Can you work these out from the model? Positions are in its coordinate system, mm. Face numbers are marked on the shaded views. A direction names the side the tool comes from. Give positions to 0.01 mm unless a question says otherwise; leave off trailing zeros. Write each loop counter-clockwise with the first axis right and the second up, starting at its lowest first coordinate (ties: lowest second). Pieces come first, ordered by that corner, then holes. Notation, with made-up numbers: M 18,35 L 39,35 A30 ccw 39,60 Z; hole C -18.75,38.25 d3. An arc over 180 degrees is marked long. Write each question's results on one line, items separated by ' | '.
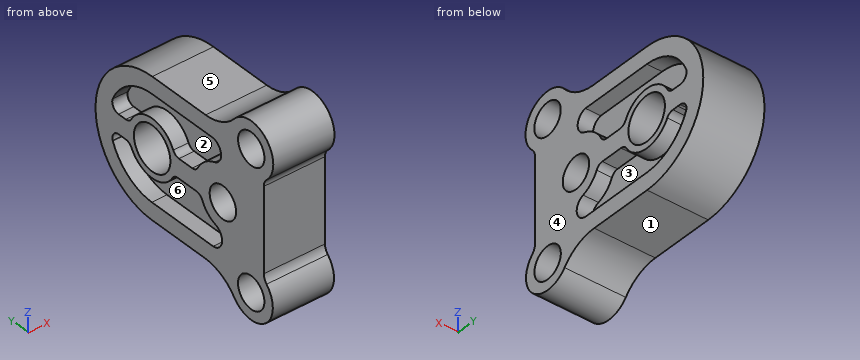
Autodesk Inventor part; units mm, degrees
ref_plane "YZ Plane" through (0, 0, 0) normal (1, 0, 0) x (0, 1, 0)
ref_plane "XZ Plane" through (0, 0, 0) normal (0, 1, 0) x (-1, 0, 0)
ref_plane "XY Plane" through (0, 0, 0) normal (0, 0, 1) x (1, 0, 0)
sketch "Sketch1" plane through (0, 0, 0) normal (1, 0, 0) x (0, 1, 0)
  arc A0 (176.1097, -208.7052) -> (175.3048, -28.7073) centre (175.5363, -118.707) ccw
  line L0 (175.3048, -28.7073) -> (90.5303, -28.7073)
  line L1 (-1.9186, -65.845) -> (-1.9186, -175.1547)
  line L2 (92.0444, -208.7052) -> (176.1097, -208.7052)
  arc A1 (44.7113, -7.4451) -> (-6.4479, -55.1041) centre (17.9836, -30.0422) ccw
  arc A2 (-6.3181, -185.8489) -> (45.0423, -231.4117) centre (18.1097, -210.0421) ccw
  line L3 (175.7375, -50.7073) -> (78.1247, -50.7073)
  line L4 (133.0218, -107.5228) -> (111.9726, -107.5228)
  line L5 (105.0926, -132.5228) -> (134.6019, -132.5228)
  arc A3 (208.5623, -100.9438) -> (141.9722, -101.9826) centre (175.5363, -118.707) ccw
  arc A4 (103.0885, -102.1131) -> (76.4229, -79.7842) centre (63.1097, -122.7698) ccw
  arc A5 (74.6044, -157.3047) -> (96.0441, -138.2655) centre (63.1097, -122.7698) ccw
  circle A6 centre (63.1097, -122.7698) radius 21
  circle A7 centre (17.9836, -30.0422) radius 21
  circle A8 centre (18.1097, -210.0421) radius 21
  arc A9 (44.7113, -7.4451) -> (90.5303, -28.7073) centre (90.5303, 31.2927) ccw
  arc A10 (92.0444, -208.7052) -> (45.0423, -231.4117) centre (92.0444, -268.7052) ccw
  arc A11 (-1.9186, -65.845) -> (-6.4479, -55.1041) centre (-16.9186, -65.845) ccw
  arc A12 (-6.3181, -185.8489) -> (-1.9186, -175.1547) centre (-17.1159, -175.1547) ccw
  arc A13 (78.1247, -50.7073) -> (76.4229, -79.7842) centre (80.8606, -65.4557) ccw
  arc A14 (74.6044, -157.3047) -> (78.6837, -186.5226) centre (79.3415, -171.5371) ccw
  circle A15 centre (175.5363, -118.707) radius 29
  arc A16 (133.0218, -107.5228) -> (141.9722, -101.9826) centre (133.0218, -97.5228) ccw
  arc A17 (143.2454, -137.4939) -> (134.6019, -132.5228) centre (134.6019, -142.5228) ccw
  arc A18 (103.0885, -102.1131) -> (111.9726, -107.5228) centre (111.9726, -97.5228) ccw
  arc A19 (105.0926, -132.5228) -> (96.0441, -138.2655) centre (105.0926, -142.5228) ccw
  line L6 (217.3693, -106.207) -> (225.3783, -106.207)
  line L7 (225.3783, -106.207) -> (229.2504, -106.207)
  line L8 (225.1161, -131.2646) -> (228.7337, -131.2481)
  line L9 (228.7337, -131.2481) -> (217.1089, -131.3029)
  arc A20 (217.1089, -131.3029) -> (208.3269, -136.6074) centre (217.156, -141.3028) ccw
  arc A21 (208.5623, -100.9438) -> (217.3693, -106.207) centre (217.3693, -96.207) ccw
  line L10 (119.8472, -132.5228) -> (119.8472, -186.8276)
  arc A22 (176.0639, -186.5226) -> (238.0141, -145.0843) centre (175.5363, -118.707) ccw
  arc A23 (143.2454, -137.4939) -> (208.3269, -136.6074) centre (175.5363, -118.707) ccw
  line L11 (176.0639, -186.5226) -> (78.6837, -186.5226)
  arc A24 (238.2111, -92.3277) -> (175.7375, -50.7073) centre (175.5363, -118.707) ccw
  line L12 (229.2504, -106.207) -> (228.9942, -106.207)
  arc A25 (228.9942, -106.207) -> (238.2111, -92.3277) centre (228.9942, -96.207) ccw
  line L13 (228.7337, -131.2481) -> (228.7379, -131.2481)
  line L14 (238.2764, -144.2509) -> (238.0141, -145.0843)
  arc A26 (238.2764, -144.2509) -> (228.7379, -131.2481) centre (228.7379, -141.2481) ccw
  point P0 (0, 0)
  point P1 (0, 0)
  point P2 (-1.9186, -182.0976)
  point P3 (139.7429, -107.5228)
  point P4 (140.8602, -132.5228)
  point P5 (105.4479, -107.5228)
  point P6 (98.1763, -132.5228)
  point P7 (-1.9186, -58.8329)
  point P8 (210.8916, -106.207)
  point P9 (242.3775, -106.207)
  dimension "d36" = 60
  dimension "d37" = 42
  dimension "d38" = 35
  dimension "d40" = 42
  dimension "d41" = 45
  dimension "d42" = 45
  dimension "d50" = 90
  dimension "d51" = 15
  dimension "d52" = 15
  dimension "d53" = 15
  dimension "d54" = 180
  dimension "d55" = 60
  dimension "d64" = 58
  dimension "d66" = 25
  dimension "d68" = 10
  dimension "d69" = 37.5
  dimension "d75" = 22
  dimension "d79" = 10
extrude "Extrusion1" add sketch "Sketch1" along normal blind 40 and the other way blind 40
sketch "Sketch2" plane through (40, 0, 0) normal (1, 0, 0) x (0, 0, -1)
  point P0 (0, 0)
extrude "Extrusion2" add sketch "Sketch1" along normal blind 20 and the other way blind 20 contours A24 A25 L7 L6 A21 A3 A16 L4 A18 A4 A13 L3 | L5 L10 L11 A14 A5 A19 | L5 A17 A23 A20 L9 L8 L13 A26 L14 A22 L11 L10
properties part number "hw1"
Item 1: I want a section at A-A, the plane y = 27.5. Please give me the cut outline in (x, z), and give its area (3 significant figures).
Geometry says:
outline: M -40,-243.12 L 40,-243.12 L 40,-228.83 L -40,-228.83 Z; M -40,-191.26 L 40,-191.26 L 40,-48.76 L -40,-48.76 Z; M -40,-11.32 L 40,-11.32 L 40,3.64 L -40,3.64 Z | area: 13,700 mm2
Item 2: I want a section at B-B, the plane z = -76. Please give me the cut outline in (x, y).
Geometry says:
outline: M -40,-1.92 L 40,-1.92 L 40,70.19 L 20,70.19 L 20,228.45 L 40,228.45 L 40,254.76 L -40,254.76 L -40,228.45 L -20,228.45 L -20,70.19 L -40,70.19 Z
Item 3: I want a section at D-D, the plane x = 15. Please give me the cut outline in (y, z) (3 decimals), and give its area (3 significant figures).
Geometry says:
outline: M -6.448,-55.104 A15.001 cw -1.919,-65.845 L -1.919,-175.155 A15.197 cw -6.318,-185.849 A34.381 ccw long 45.042,-231.412 A60 cw 92.044,-208.705 L 176.11,-208.705 A90 ccw 175.305,-28.707 L 90.53,-28.707 A60 cw 44.711,-7.445 A35 ccw long Z; hole C 17.984,-30.042 d42; hole C 18.11,-210.042 d42; hole C 63.11,-122.77 d42; hole C 175.536,-118.707 d58 | area: 42,600 mm2
Item 4: I'm going to push flat-ended pins straight in: pin 1 (1 mm diameter, centred on x = 25.5, y = 13, fed in from +Z); pin 2 (6 mm diameter, centred on x = -33.5, y = 222, fed in from +Z); pin 3 (6 mm diameter, centred on x = -29, y = 123.5, fed in from +Z); pin 4 (25 mm diameter, centred on y = 17.98, z = -30.04, fed in from -X). Where does each tip first touch, or does it pass through?
Geometry says:
pin 1: stops at z = 4.67 | pin 2: stops at z = -39.9 | pin 3: stops at z = -28.71 | pin 4: passes through
Item 5: If I drill on line 1 (Z direction, x = -33.5, y = 112.5); line 2 (Z direction, x = -1, y = 8.5); line 3 (Y direction, x = 31, z = -141.5), over which ranges is the centre line in solid material (lowest first)? Write a range as from..to.
Geometry says:
line 1: z = -208.71..-186.52, -132.52..-107.52, -50.71..-28.71 | line 2: z = -243.05..-228.71, -191.37..-48.78, -11.31..3.65 | line 3: y = -1.92..53.61, 72.61..94.32, 145.94..157.61, 193.47..205.14, 238.73..262.6
Item 6: I want a section at C-C, the plane y = 120.5. Please give me the cut outline in (x, z).
Geometry says:
outline: M -40,-208.71 L 40,-208.71 L 40,-186.52 L 20,-186.52 L 20,-132.52 L 40,-132.52 L 40,-107.52 L 20,-107.52 L 20,-50.71 L 40,-50.71 L 40,-28.71 L -40,-28.71 L -40,-50.71 L -20,-50.71 L -20,-107.52 L -40,-107.52 L -40,-132.52 L -20,-132.52 L -20,-186.52 L -40,-186.52 Z
Item 7: For the marked faces 1, 2 and 3, which set-ups out of +Z, -Z, +X, -X, +Y, -Y let a thin tool reach every point of the face, with its end or its side?
Geometry says:
face 1: -Z, +X, -X, +Y | face 2: -X | face 3: +X
Item 8: Thinking about a two-plate mould opening in Z: for the marked faces 4, 5 and 6, which applies, +Z half, -Z half, draft (parallel to the pull), parting line (faces both ways), or undercut?
Geometry says:
face 4: draft | face 5: +Z half | face 6: undercut
